from build123d import *

# Parameters (mm, degrees)
F0_W     = 100
F0_H     = 100
F1_DEPTH = 20
F2_R     = 25
F3_DEPTH = 10
F4_W     = 70
F4_H     = 70
F5_DEPTH = 5


with BuildPart() as f1:
    # F0 (on Top) → F1 (new body)
    with BuildSketch(Plane.XY):
        Rectangle(F0_W, F0_H)
    extrude(amount=F1_DEPTH)

    # F2 (on face) → F3 (cut)
    with BuildSketch(Plane.XY.offset(20)):
        with Locations((-2.75913, 0)):
            Circle(F2_R)
    extrude(amount=-F3_DEPTH, mode=Mode.SUBTRACT)

    # F4 (on face) → F5 (cut)
    with BuildSketch(Plane.XY.offset(20)):
        Rectangle(F4_W, F4_H)
    extrude(amount=-F5_DEPTH, mode=Mode.SUBTRACT)


solid = f1.part
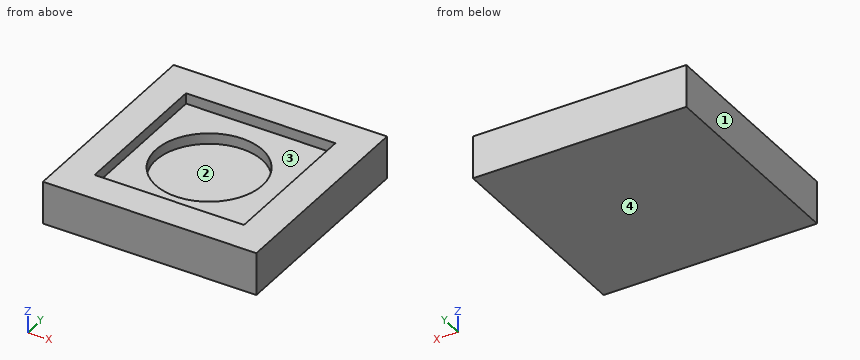
Can you work these out from the model? Positions are in its coordinate system, mm. Face numbers are marked on the shaded views. Coordinates: 2 decimals unless noted, no trailing zeros. Loops run counter-clockwise (first coordinate to the right, second up) from the corner with the lowest first, then second, coordinate; pieces in that order, holes last. Notation, with made-up numbers: (-28, 83.5) - (7, 83.5) arc R15 cw to (7, 104.5) - close; hole circle Ø4 at (69.5, 65). An arc over 180 degrees is marked (long way). Answer as a JSON object with one key per item and string values. Group by question number.
Item 1: If we mould it in two halves opening along X, with no side actions, what happens to the marked faces 1, 2, 3 and 4? For each: released by +X, released by -X, zero draft, split by the parting line, or undercut.
Item 2: If I drill on L1, parallel to Y at x = 26.5, z = 17.5; L2, parallel to Z at x = 14.5, y = -32.5, over which ranges is the centre line in solid material (lowest first)? Write a range as from..to.
Item 3: If we section it at B-B (x = -1): List the corners of the cut face in (y, z) for me, plus the area to 3 significant figures.
Item 4: If we section it at D-D (y = 12.5): List the corners of the cut face in (x, z) for me.
Item 5: For pin 1 (4 mm diameter, centred on x = -15.5, y = -18.5, fed in from +Z); pin 2 (10 mm diameter, centred on x = 7, y = 26.5, fed in from +Z), each with a flat end and sliding along its axis, tell me the tip position at first contact or that it passes through.
Item 6: If we section it at C-C (z = 13): List the corners of the cut face in (x, y) for me, plus the area to 3 significant figures.
Item 7: If we section it at A-A (y = -30): List the corners of the cut face in (x, z) for me.
Returned:
{
 "1": {"face 1": "released by -X", "face 2": "undercut", "face 3": "undercut", "face 4": "zero draft"},
 "2": {"L1": "y = -50..-35, 35..50", "L2": "z = 0..15"},
 "3": {"outline": "(-50, 0) - (50, 0) - (50, 20) - (35, 20) - (35, 15) - (24.94, 15) - (24.94, 10) - (-24.94, 10) - (-24.94, 15) - (-35, 15) - (-35, 20) - (-50, 20) - close", "area": "1,400 mm²"},
 "4": {"outline": "(-50, 0) - (50, 0) - (50, 20) - (35, 20) - (35, 15) - (18.89, 15) - (18.89, 10) - (-24.41, 10) - (-24.41, 15) - (-35, 15) - (-35, 20) - (-50, 20) - close"},
 "5": {"pin 1": "stops at z = 10", "pin 2": "stops at z = 15"},
 "6": {"outline": "(-50, -50) - (50, -50) - (50, 50) - (-50, 50) - close; hole circle Ø50 at (-2.76, 0)", "area": "8,040 mm²"},
 "7": {"outline": "(-50, 0) - (50, 0) - (50, 20) - (35, 20) - (35, 15) - (-35, 15) - (-35, 20) - (-50, 20) - close"}
}
